Can you work these out from the model? Positions are in its coordinate system, mm. Give positions to 0.01 mm unless a question says otherwise; leave off trailing zeros. Loops run counter-clockwise (first coordinate to the right, second up) from the corner with the lowest first, then second, coordinate; pieces in that order, holes last. Notation, with made-up numbers: M -16,-11.5 L 11,-11.5 A37 cw 11,24.5 Z; hole C 87,-27.75 d1. An arc over 180 degrees is marked long. Put each result on its own line as item: value. Start each with the question number.
1) Imagine slicing it at D-D (z = 15). Write out the boundary of the cut face in (x, y).
2) For P1, Ø1, axis at y = -6.5, z = 23, coming from the -X side; P2, Ø4, axis at x = 15.5, y = -15, coming from the +Z side; P3, Ø6, axis at y = 14, z = 5.5, coming from the +X side; P4, Ø1, axis at x = -5.5, y = -10, coming from the +Z side, each with a flat end and sliding along its axis, tell me the tip position at first contact or that it passes through.
3) Please list where these lines run through material, in increasing order: line 1 along Y through (x, z) = (5, 7); line 2 along Z through (x, y) = (0, 10); line 3 along X through (y, z) = (-12, 5.5). Write a range as from..to.
4) Imagine slicing it at A-A (z = 6.75). Write out the boundary of the cut face in (x, y), then the cut area to 3 significant figures.
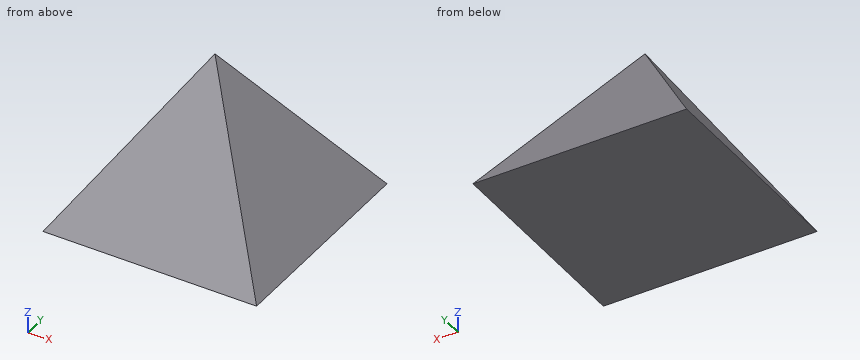
from build123d import *

# Parameters (mm, degrees)
F0_W     = 40
F0_H     = 40
F1_DEPTH = 30
F2_SIZE2 = 29.99999
F2_SIZE  = 19.99999


# Not quite as in the source:
# - a fillet or chamfer is up to 0.001 mm smaller than in the source, because OpenCascade refuses the exact size


with BuildPart() as f1:
    # F0 (on Top) → F1 (new body)
    with BuildSketch(Plane.XY):
        Rectangle(F0_W, F0_H)
    extrude(amount=F1_DEPTH)

    # F2 (size 20 and 30 in the source; OpenCascade refuses exactly that, so slightly less here)
    f2_edges = [f1.edges().sort_by_distance(p)[0] for p in [
        (-20, 0, 30),
        (0, 20, 30),
        (0, -20, 30),
        (20, 0, 30),
    ]]
    f2_side = f1.faces().sort_by_distance((0, 0, 30))[0]
    chamfer(f2_edges, length=F2_SIZE, length2=F2_SIZE2, reference=f2_side)


solid = f1.part
Recorded:
1. outline: M -10,-10 L 10,-10 L 10,10 L -10,10 Z
2. P1: through
2. P2: z = 9.21
2. P3: x = 18.33
2. P4: z = 15.75
3. line 1: -15.33..15.33
3. line 2: 0..15
3. line 3: -16.33..16.33
4. outline: M -15.5,-15.5 L 15.5,-15.5 L 15.5,15.5 L -15.5,15.5 Z
4. area: 961 mm²
